Input: part model. Units: mm. Frame: model coordinates. Face numbers are marked on the shaded views. A direction names the side the tool comes from. Coordinates: 2 decimals unless noted, no trailing zeros. Order: outer loops, then holes, each group sorted by start corner. A loop starts at its lowest first (then second) coordinate and runs counter-clockwise, first axis right, second up. Notation, with made-up numbers: M 59.5,-29 L 98.5,-29 A28 ccw 98.5,-10 Z; hole C -4.75,10.5 d11. An arc over 180 degrees is marked long. Answer in a Markdown table with one row per item.
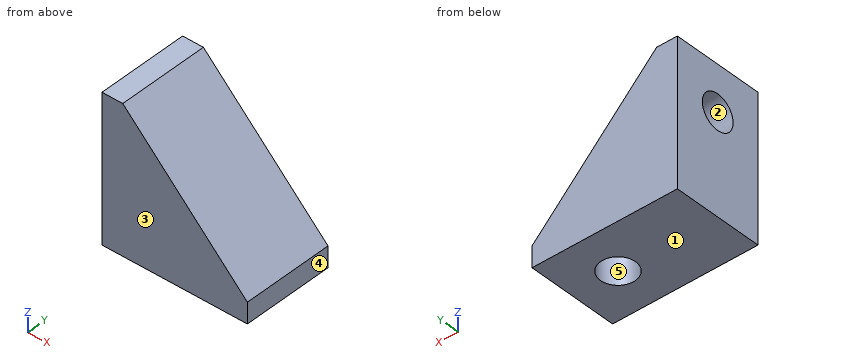
Autodesk Inventor part; units mm, degrees
ref_plane "YZ Plane" through (0, 0, 0) normal (1, 0, 0) x (0, 1, 0)
ref_plane "XZ Plane" through (0, 0, 0) normal (0, 1, 0) x (-1, 0, 0)
ref_plane "XY Plane" through (0, 0, 0) normal (0, 0, 1) x (1, 0, 0)
sketch "Boceto1" plane through (0, 0, 0) normal (0, 0, 1) x (1, 0, 0)
  circle A0 centre (88, 48.5) radius 1.5
  circle A1 centre (88, -51.5) radius 1.5
  circle A2 centre (-50, 86.5) radius 1.5
  circle A3 centre (50, 86.5) radius 1.5
  circle A4 centre (-88, -51.5) radius 1.5
  circle A5 centre (-88, 48.5) radius 1.5
  circle A6 centre (50, -89.5) radius 1.5
  circle A7 centre (-50, -89.5) radius 1.5
  line L0 (-103, -104.5) -> (-103, 101.5)
  line L1 (103, -104.5) -> (-103, -104.5)
  line L2 (103, 101.5) -> (103, -104.5)
  line L3 (-100, -104.5) -> (-100, 89.3)
  line L4 (-88, -51.5) -> (-100, -51.5)
  line L5 (-88, -51.5) -> (-82.5, -51.5)
  line L6 (-82.5, -51.5) -> (-82.5, -57)
  line L7 (-82.5, -57) -> (-100, -57)
  line L8 (-100, -57) -> (-100, -46)
  line L9 (-100, -46) -> (-82.5, -46)
  line L10 (-82.5, -46) -> (-82.5, -57)
  circle A8 centre (-88, -51.5) radius 2.1
  line L11 (-103, 101.5) -> (103, 101.5)
  point P0 (0, 0)
  dimension "d0" = 5.5
  dimension "d1" = 5.5
  dimension "d2" = 11
  dimension "d14" = 4.2
extrude "Extrusión1" add sketch "Boceto1" along normal blind 17.5 contours L5 L4 A4 | L5 A8 L4 A4 | A4 L4 L5 | A4 L4 A8 L5 | A8 L4 L3 L9 L10 L5 | L5 L6 L7 L3 L4 A8
sketch "Boceto2" plane through (-100, -57, 0) normal (-1, 0, 0) x (0, 0, 1)
  line L0 (0, 0) -> (17.5, 0)
  line L1 (0, 11) -> (0, 0)
  point P0 (0, 57)
  point P1 (12, 5.5)
  dimension "d5" = 5.5
  dimension "d6" = 12
hole "Agujero1" at (-100, -51.5, 12) direction (1, 0, 0) diameter 4.2 depth 4
sketch "Boceto3" plane through (0, 0, 0) normal (0, 0, -1) x (-1, 0, 0)
  line L0 (100, -46) -> (100, -57)
  line L1 (82.5, -46) -> (100, -46)
  point P0 (0, 0)
  point P1 (88, -51.5)
  dimension "d15" = 12
  dimension "d16" = 5.5
hole "Agujero2" at (-88, -51.5, 0) direction (0, 0, 1) diameter 4.2 depth 4
chamfer "Chaflán1" distance 15 angle 45 1 edges at (-82.5, -51.5, 17.5)
properties part number "Union_Inferior"
1) Reachability of the marked faces 1 and 2 from +Z, -Z, +X, -X, +Y, -Y: full face, straight path, thin tool, end or side. Return the list, or none.
Resolved:
| item | result |
|---|---|
| face 1 | -Z, +X, -X, +Y, -Y |
| face 2 | -X |
2) Contact query for flat-ended pins moving along their axis: pin 1 (3.5 mm diameter, centred on y = -51.5, z = 12, fed in from -X); pin 2 (1.5 mm diameter, centred on y = -55, z = 8.5, fed in from +X); pin 3 (4 mm diameter, centred on x = -88, y = -51.5, fed in from -Z). Output: stop coordinate, or through.
Resolved:
| item | result |
|---|---|
| pin 1 | stops at x = -96 |
| pin 2 | stops at x = -87.75 |
| pin 3 | stops at z = 4 |
3) Cut plane A-A, the plane z = 12. Output: boundary loops of the cut face in (x, y), and give its area (3 significant figures).
Resolved:
| item | result |
|---|---|
| outline | M -100,-57 L -92,-57 L -92,-46 L -100,-46 L -100,-49.4 L -96,-49.4 L -96,-53.6 L -100,-53.6 Z |
| area | 71.2 mm2 |
4) Mould query, pull axis X, two halves, no side actions, for the marked faces 3, 4 and 5. Classes: +X half, -X half, draft (parallel to the pull), parting line (faces both ways), or undercut.
Resolved:
| item | result |
|---|---|
| face 3 | draft |
| face 4 | +X half |
| face 5 | undercut |
5) Material intervals for probe 1 along Y at (x, z) = (-98.25, 12); probe 2 along X at (y, z) = (-51.5, 1.9); probe 3 along X at (y, z) = (-51.5, 2.55), sorted ascending.
Resolved:
| item | result |
|---|---|
| probe 1 | y = -57 to -53.6, -49.4 to -46 |
| probe 2 | x = -100 to -90.1, -85.9 to -82.5 |
| probe 3 | x = -100 to -90.1, -85.9 to -82.55 |
6) Cut plane C-C, the plane x = -88. Output: boundary loops of the cut face in (y, z), and give its area (3 significant figures).
Resolved:
| item | result |
|---|---|
| outline | M -57,0 L -53.6,0 L -53.6,4 L -49.4,4 L -49.4,0 L -46,0 L -46,8 L -57,8 Z |
| area | 71.2 mm2 |
7) Cut plane D-D, the plane z = 3.25. Output: boundary loops of the cut face in (x, y), and give its area (3 significant figures).
Resolved:
| item | result |
|---|---|
| outline | M -100,-57 L -83.25,-57 L -83.25,-46 L -100,-46 Z; hole C -88,-51.5 d4.2 |
| area | 170 mm2 |
8) Cut plane B-B, the plane y = -51.5. Output: boundary loops of the cut face in (x, z).
Resolved:
| item | result |
|---|---|
| outline | M -100,0 L -90.1,0 L -90.1,4 L -85.9,4 L -85.9,0 L -82.5,0 L -82.5,2.5 L -97.5,17.5 L -100,17.5 L -100,14.1 L -96,14.1 L -96,9.9 L -100,9.9 Z |
